Autodesk Inventor part; units mm, degrees
ref_plane "YZ Plane" through (0, 0, 0) normal (1, 0, 0) x (0, 1, 0)
ref_plane "XZ Plane" through (0, 0, 0) normal (0, 1, 0) x (-1, 0, 0)
ref_plane "XY Plane" through (0, 0, 0) normal (0, 0, 1) x (1, 0, 0)
sketch "Sketch1" plane through (0, 0, 0) normal (0, 1, 0) x (-1, 0, 0)
  circle A0 centre (0, 0) radius 20
  circle A1 centre (0, 0) radius 6
  dimension "d0" = 40
  dimension "d1" = 12
extrude "Extrusion1" add sketch "Sketch1" along normal blind 3
sketch "Sketch2" plane through (0, 3, 0) normal (0, 1, 0) x (1, 0, 0)
  circle A0 centre (0, 0) radius 7.5
  point P0 (-7.5, 0)
  dimension "d4" = 15
hole "Hole1" at (-7.5, 3, 0) direction (0, -1, 0) diameter 2.2 end through all
pattern_circular "Circular Pattern1" count 4 over 360 about axis through (0, 0, 0) along (0, 1, 0) of "Hole1"
sketch "Sketch4" plane through (0, 3, 0) normal (0, 1, 0) x (1, 0, 0)
  line L0 (0, 0) -> (13, 0)
  dimension "d27" = 13
hole "Hole3" at (13, 3, 0) direction (0, -1, 0) diameter 2.2 end through all
pattern_circular "Circular Pattern3" count 4 over 360 about axis through (0, 0, 0) along (0, 1, 0) of "Hole3"
properties part number "back2"
The listing builds one solid part. Answer for the finished solid, in the listing's coordinates (mm). Give positions to 0.01 mm unless a question says otherwise; leave off trailing zeros. Order: outer loops, then holes, each group sorted by start corner. A loop starts at its lowest first (then second) coordinate and runs counter-clockwise, first axis right, second up. Notation, with made-up numbers: (-29, 26.25) -> (27, 26.25) arc R27 ccw to (27, 53.25) -> close; hole circle Ø11 at (77.5, 88). An arc over 180 degrees is marked (long way). Put each result on its own line as item: value.
Item 1: Given P1, Ø1, axis at x = -12, y = 0.5, coming from the +Z side, flat-ended and moving along its own axis, determine where the tip first touches the part or whether it passes through.
Established:
P1: stops at z = 16.36
Item 2: A cutting plane is placed at A-A on x = 0. Give the vertices of the cut face in (y, z), plus the area to 3 significant figures.
Established:
outline: (0, -20) -> (3, -20) -> (3, -14.1) -> (0, -14.1) -> close; (0, -11.9) -> (3, -11.9) -> (3, -8.6) -> (0, -8.6) -> close; (0, -6.4) -> (3, -6.4) -> (3, -6) -> (0, -6) -> close; (0, 6) -> (3, 6) -> (3, 6.4) -> (0, 6.4) -> close; (0, 8.6) -> (3, 8.6) -> (3, 11.9) -> (0, 11.9) -> close; (0, 14.1) -> (3, 14.1) -> (3, 20) -> (0, 20) -> close
area: 57.6 mm^2
Item 3: For a pull along Z with two mould halves and no side action, classify faces 1 (the face through (-4, 3, 5)), 2 (the face through (4.336, 1.479, 19.524)), 3 (the face through (-0.238, 1.479, -14.074)) as released by +Z, released by -Z, zero draft, split by the parting line, or undercut.
Established:
face 1: zero draft
face 2: split by the parting line
face 3: undercut
Item 4: A cutting plane is placed at D-D on x = -13. Give the vertices of the cut face in (y, z).
Established:
outline: (0, -15.2) -> (3, -15.2) -> (3, -1.1) -> (0, -1.1) -> close; (0, 1.1) -> (3, 1.1) -> (3, 15.2) -> (0, 15.2) -> close
Item 5: Straight lines are drawn through the part: line 1 (Z direction, x = 0, y = 1.65); line 2 (Z direction, x = -1, y = 2.1); line 3 (Z direction, x = 4, y = 1.85). For each, find the intervals that lie inside material, in ascending order.
Established:
line 1: z = -20 to -14.1, -11.9 to -8.6, -6.4 to -6, 6 to 6.4, 8.6 to 11.9, 14.1 to 20
line 2: z = -19.97 to -13.46, -12.54 to -7.96, -7.04 to -5.92, 5.92 to 7.04, 7.96 to 12.54, 13.46 to 19.97
line 3: z = -19.6 to -4.47, 4.47 to 19.6
Item 6: A cutting plane is placed at B-B on z = 13. Give the vertices of the cut face in (x, y), plus the area to 3 significant figures.
Established:
outline: (-15.2, 0) -> (-1.1, 0) -> (-1.1, 3) -> (-15.2, 3) -> close; (1.1, 0) -> (15.2, 0) -> (15.2, 3) -> (1.1, 3) -> close
area: 84.6 mm^2
Item 7: A cutting plane is placed at C-C on y = 2.1. Count the separate pieces of the cut face and the enclosed holes in it, plus the area to 3 significant figures.
Established:
separate pieces: 1
enclosed holes: 9
area: 1,110 mm^2
